Could you check a few things on this model? Use its own coordinates, in mm. Face numbers are marked on the shaded views. A direction names the side the tool comes from. Give positions to 0.01 mm unless a question says otherwise; leave off trailing zeros. Write each loop counter-clockwise with the first axis right and the second up, starting at its lowest first coordinate (ties: lowest second). Pieces come first, ordered by that corner, then holes. Notation, with made-up numbers: (24.25, 87.5) - (28.25, 87.5) arc R30 cw to (28.25, 118.5) - close; hole circle Ø3 at (62, -4.5). An arc over 180 degrees is marked (long way). Answer in a Markdown table with one row per item.
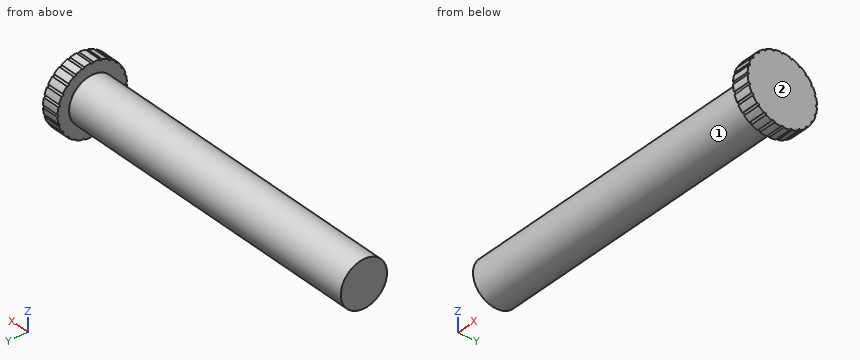
from build123d import *

# Parameters (mm, degrees)
SKETCH1_R           = 4
BOSS_EXTRUDE2_DEPTH = 55.94
SKETCH2_R           = 6
BOSS_EXTRUDE3_DEPTH = 3
SKETCH3_R           = 0.2
CUT_EXTRUDE1_DEPTH  = 3
CIRPATTERN1_COUNT   = 24


with BuildPart() as part:
    # Sketch1 → Boss-Extrude2 (new body)
    with BuildSketch(Plane(origin=(0, 0, 0), x_dir=(0, 0, -1), z_dir=(1, 0, 0))):
        Circle(SKETCH1_R)
    extrude(amount=BOSS_EXTRUDE2_DEPTH)

    # Sketch2 → Boss-Extrude3 (add)
    with BuildSketch(Plane(origin=(55.94, 0, 0), x_dir=(0, 0, -1), z_dir=(1, 0, 0))):
        Circle(SKETCH2_R)
    extrude(amount=BOSS_EXTRUDE3_DEPTH)

    # Sketch3 → Cut-Extrude1 (cut)
    with BuildSketch(Plane(origin=(58.94, 0, 0), x_dir=(0, 0, -1), z_dir=(1, 0, 0))):
        with Locations((-6, 0)):
            Circle(SKETCH3_R)
    cut_extrude1 = extrude(amount=-CUT_EXTRUDE1_DEPTH, mode=Mode.SUBTRACT)

    # CirPattern1: Cut-Extrude1 ×24 about axis
    cirpattern1_axis = Axis((0, 0, -0.003264402), (1, 0, 0))
    for i in range(1, CIRPATTERN1_COUNT):
        add(cut_extrude1.rotate(cirpattern1_axis, i * 360 / CIRPATTERN1_COUNT), mode=Mode.SUBTRACT)


solid = part.part
1) Imagine slicing it at A-A (x = 38). List the corners of the cut face in (y, z) for me, then the cut area to 3 significant figures.
Check values:
| item | result |
|---|---|
| outline | circle Ø8 at (0, 0) |
| area | 50.3 mm2 |
2) Imagine slicing it at B-B (z = 0.75). List the corners of the cut face in (x, y) for me, then the cut area to 3 significant figures.
Check values:
| item | result |
|---|---|
| outline | (0, -3.93) - (55.94, -3.93) - (55.94, -5.95) - (58.94, -5.95) - (58.94, 5.95) - (55.94, 5.95) - (55.94, 3.93) - (0, 3.93) - close |
| area | 475 mm2 |
3) Will these pins go through, and if not, where does the flat tip stop? P1, Ø1.5, axis at x = 33, y = 3, coming from the -Z side; P2, Ø3, axis at x = 47.5, y = 2.5, coming from the -Z side; P3, Ø6, axis at x = 25.5, y = -1.5, coming from the +Z side.
Check values:
| item | result |
|---|---|
| P1 | stops at z = -3.31 |
| P2 | stops at z = -3.87 |
| P3 | stops at z = 4 |
4) On a 3-axis mill with a long thin cutter (end or side, diameter ignored), from which of +Z, -Z, +X, -X, +Y, -Y can I reach the whole of each face in a straight line? I mean the marked faces 1 and 2. Say none if no direction works.
Check values:
| item | result |
|---|---|
| face 1 | -X |
| face 2 | +Z, -Z, +X, +Y, -Y |
5) If I drill on line 1 (Z direction, x = 54.5, y = -0.25); line 2 (X direction, y = 3.75, z = 1.75); line 3 (Y direction, x = 50.5, z = -1), over which ranges is the centre line in solid material (lowest first)?
Check values:
| item | result |
|---|---|
| line 1 | z = -3.99 to 3.99 |
| line 2 | x = 55.94 to 58.94 |
| line 3 | y = -3.87 to 3.87 |
